Read the model definition and answer for the solid it produces. Units are mm, in the model's axes. A direction names the side the tool comes from. Round coordinates to 2 decimals unless told otherwise and drop trailing zeros. Write each loop counter-clockwise with the first axis right and the second up, starting at its lowest first coordinate (ties: lowest second). Pieces come first, ordered by that corner, then holes. Notation, with made-up numbers: (-30, -30) - (-26, -30) arc R13 cw to (-26, -26) - close; hole circle Ø3 at (-12, -39). An arc over 180 degrees is marked (long way). Answer as CSV lines item,"result". Start each with the question number.
1) For a pull along X with two mould halves and no side action, classify faces 5 (the cylindrical face through (39.34, 291.3, 1.48)), 6 (the flat face through (20, 263.848, 1)), 7 (the flat face through (69.182, 249.677, 1.479)), 8 (the cylindrical face through (76.194, 254.669, 1.479)) as +X half, -X half, draft (parallel to the pull), parting line (faces both ways), or undercut.
2) Each of these flat-tipped pins is pushed along its axis until it touches: pin 1 (0.9 mm diameter, centred on x = 47, z = 1, fed in from -Y); pin 2 (2.5 mm diameter, centred on x = 55.89, y = 264.68, fed in from -Z); pin 3 (1 mm diameter, centred on y = 246.5, z = 0.5, fed in from -X); pin 4 (1.5 mm diameter, centred on y = 262, z = 2, fed in from +X). Where does it stop, or does it pass through?
3) Find section A-A on z = 1.7. State how many separate pieces and enclosed holes the cut face has, then the cut area to 3 significant figures.
4) Find section B-B on y = 244. Determine the outline of the cut face in (x, z), then the cut area to 3 significant figures.
5) Consider line 1 along Y through (x, z) = (47, 2.6); line 2 along X through (y, z) = (262, 1.15); line 3 along Y through (x, z) = (34.5, 2.15). Determine where each line is inside the solid, lowest interval first.
6) Which of the six approach directions +Z, -Z, +X, -X, +Y, -Y give full straight-line access (tool end or side, diameter ignored) to faces 1 (the flat face through (70.38, 247.23, 1.48)), 2 (the flat face through (45.694, 235, 1)), 3 (the flat face through (23.953, 247.198, 1.479)), 4 (the flat face through (62.31, 285.53, 1.48))?
7) Find section C-C on x = 62. Determine the outline of the cut face in (y, z).
from build123d import *

# Parameters (mm, degrees)
MODEL_R                 = 1.5
MODEL_R_2               = 2
SALIENTE_EXTRUIR1_DEPTH = 3


with BuildPart() as part:
    # Model → Saliente-Extruir1 (new body)
    with BuildSketch(Plane.XY):
        with BuildLine():
            Line((61.181496903, 283.575359896), (63.474021053, 287.546128202))
            ThreePointArc((63.474021053, 287.546128202), (68.406948117, 283.561065799), (72.392010519, 278.628138736))
            Line((72.392010519, 278.628138736), (68.421242213, 276.335614586))
            Line((68.421242213, 276.335614586), (69.921242213, 273.737538374))
            Line((69.921242213, 273.737538374), (73.892010519, 276.030062525))
            ThreePointArc((73.892010519, 276.030062525), (76.17151947, 270.112433717), (77.156221214, 263.847862364))
            Line((77.156221214, 263.847862364), (72.571172914, 263.847862364))
            Line((72.571172914, 263.847862364), (72.571172914, 260.847862364))
            Line((72.571172914, 260.847862364), (77.156221214, 260.847862364))
            ThreePointArc((77.156221214, 260.847862364), (76.17151947, 254.583291011), (73.892010519, 248.665662203))
            Line((73.892010519, 248.665662203), (69.921242213, 250.958186353))
            Line((69.921242213, 250.958186353), (68.421242213, 248.360110142))
            Line((68.421242213, 248.360110142), (72.392010519, 246.067585992))
            ThreePointArc((72.392010519, 246.067585992), (68.406948117, 241.134658928), (63.474021053, 237.149596526))
            Line((63.474021053, 237.149596526), (61.181496903, 241.120364831))
            Line((61.181496903, 241.120364831), (58.583420692, 239.620364831))
            Line((58.583420692, 239.620364831), (60.875944842, 235.649596526))
            ThreePointArc((60.875944842, 235.649596526), (54.958316034, 233.370087575), (48.693744681, 232.385385831))
            Line((48.693744681, 232.385385831), (48.693744681, 236.970434131))
            Line((48.693744681, 236.970434131), (45.693744681, 236.970434131))
            Line((45.693744681, 236.970434131), (45.693744681, 232.385385831))
            ThreePointArc((45.693744681, 232.385385831), (39.429173328, 233.370087575), (33.51154452, 235.649596526))
            Line((33.51154452, 235.649596526), (35.80406867, 239.620364831))
            Line((35.80406867, 239.620364831), (33.205992459, 241.120364831))
            Line((33.205992459, 241.120364831), (30.913468309, 237.149596526))
            ThreePointArc((30.913468309, 237.149596526), (25.980541245, 241.134658928), (21.995478843, 246.067585992))
            Line((21.995478843, 246.067585992), (25.966247149, 248.360110142))
            Line((25.966247149, 248.360110142), (24.466247149, 250.958186353))
            Line((24.466247149, 250.958186353), (20.495478843, 248.665662203))
            ThreePointArc((20.495478843, 248.665662203), (18.215969892, 254.583291011), (17.231268148, 260.847862364))
            Line((17.231268148, 260.847862364), (21.816316448, 260.847862364))
            Line((21.816316448, 260.847862364), (21.816316448, 263.847862364))
            Line((21.816316448, 263.847862364), (17.231268148, 263.847862364))
            ThreePointArc((17.231268148, 263.847862364), (18.215969892, 270.112433717), (20.495478843, 276.030062525))
            Line((20.495478843, 276.030062525), (24.466247149, 273.737538374))
            Line((24.466247149, 273.737538374), (25.966247149, 276.335614586))
            Line((25.966247149, 276.335614586), (21.995478843, 278.628138736))
            ThreePointArc((21.995478843, 278.628138736), (25.980541245, 283.561065799), (30.913468309, 287.546128202))
            Line((30.913468309, 287.546128202), (33.205992459, 283.575359896))
            Line((33.205992459, 283.575359896), (35.80406867, 285.075359896))
            Line((35.80406867, 285.075359896), (33.51154452, 289.046128202))
            ThreePointArc((33.51154452, 289.046128202), (39.429173328, 291.325637152), (45.693744681, 292.310338897))
            Line((45.693744681, 292.310338897), (45.693744681, 287.725290597))
            Line((45.693744681, 287.725290597), (48.693744681, 287.725290597))
            Line((48.693744681, 287.725290597), (48.693744681, 292.310338897))
            ThreePointArc((48.693744681, 292.310338897), (54.958316034, 291.325637152), (60.875944842, 289.046128202))
            Line((60.875944842, 289.046128202), (58.583420692, 285.075359896))
            Line((58.583420692, 285.075359896), (61.181496903, 283.575359896))
        make_face()
        with Locations((55.887077118, 264.67723377)):
            Circle(MODEL_R, mode=Mode.SUBTRACT)
        with Locations((38.500412244, 260.018490958)):
            Circle(MODEL_R, mode=Mode.SUBTRACT)
        with Locations((47.193744681, 262.347862364)):
            Circle(MODEL_R_2, mode=Mode.SUBTRACT)
        with Locations((44.864373275, 271.0411948)):
            Circle(MODEL_R, mode=Mode.SUBTRACT)
        with Locations((49.523116087, 253.654529927)):
            Circle(MODEL_R, mode=Mode.SUBTRACT)
    extrude(amount=SALIENTE_EXTRUIR1_DEPTH)


solid = part.part
Check values:
1,face 5,"-X half"
1,face 6,"draft"
1,face 7,"undercut"
1,face 8,"+X half"
2,pin 1,"stops at y = 236.97"
2,pin 2,"passes through"
2,pin 3,"stops at x = 22"
2,pin 4,"stops at x = 72.57"
3,separate pieces,"1"
3,enclosed holes,"5"
3,area,"2,620 mm^2"
4,outline,"(23.46, 0) - (70.93, 0) - (70.93, 3) - (23.46, 3) - close"
4,area,"142 mm^2"
5,line 1,"y = 236.97 to 260.36, 264.34 to 287.73"
5,line 2,"x = 21.82 to 45.22, 49.16 to 72.57"
5,line 3,"y = 235.17 to 237.36, 240.37 to 284.32, 287.33 to 289.53"
6,face 1,"+Z, -Z, +X"
6,face 2,"+Z, -Z, -Y"
6,face 3,"+Z, -Z, -X"
6,face 4,"+Z, -Z, +Y"
7,outline,"(239.7, 0) - (284.99, 0) - (284.99, 3) - (239.7, 3) - close"
